Read the model definition and answer for the solid it produces. Units are mm, in the model's axes. Face numbers are marked on the shaded views. Give positions to 0.01 mm unless a question says otherwise; leave off trailing zeros. Put each result on its own line as item: value. Start each with the question number.
1. Given pin 1 Ø5 at (x, z) = (-13.5, -45.5) entering from +Y; pin 2 Ø10 at (x, z) = (2, -15.5) entering from -Y; pin 3 Ø1.5 at (x, y) = (-6.5, -9) entering from -Z; pin 4 Ø1 at (x, y) = (-8, -5.5) entering from -Z, each flat-ended and moving along its own axis, determine where each tip first touches the part or whether it passes through.
2. For a pull along Z with two mould halves and no side action, classify the marked faces 1, 2 and 3 as released by +Z, released by -Z, zero draft, split by the parting line, or undercut.
3. Consider L1, parallel to Z at x = 0, y = -8.5; L2, parallel to Z at x = 0, y = -1.85; L3, parallel to Z at x = 0, y = -11.25. Determine where each line is inside the solid, lowest interval first. Write a range as from..to.
4. A cutting plane is placed at A-A, the plane y = -9. Count the separate pieces of the cut face and the enclosed holes in it, plus the area to 3 significant figures.
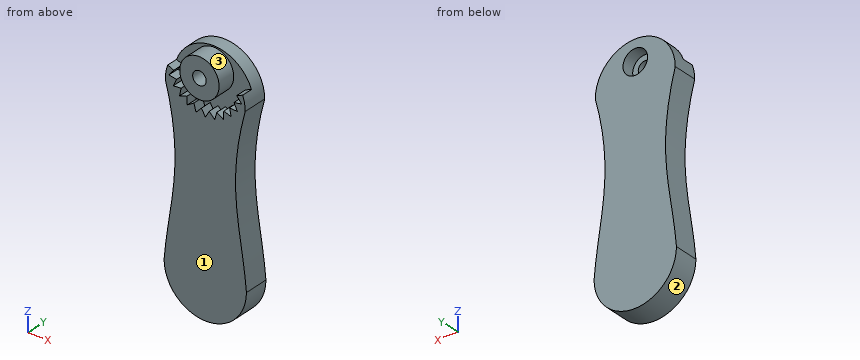
```python
from build123d import *

# Parameters (mm, degrees)
F1_DEPTH = 10.16
F2_R     = 8.128
F2_R_2   = 2.794
F3_DEPTH = 3.048
F4_DEPTH = 50.8
F5_R     = 8.128
F6_DEPTH = 4.572
F7_R     = 5.08
F7_R_2   = 2.794
F8_DEPTH = 5.08


with BuildPart() as f1:
    # F0 (on Front) → F1 (new body)
    with BuildSketch(Plane.XZ):
        with BuildLine():
            add(Edge.make_bspline(
                [(16.51, 16.2022389048), (8.1950903917, -14.7107664531), (15.1309384414, -29.2677398155), (17.018, -51.8697610952)],
                knots=[0, 0, 0, 0, 68.073895496, 68.073895496, 68.073895496, 68.073895496], degree=3))
            ThreePointArc((16.51, 16.2022389048), (0, 32.7122389048), (-16.51, 16.2022389048))
            add(Edge.make_bspline(
                [(-16.51, 16.2022389048), (-8.1950903917, -14.7107664531), (-15.1309384414, -29.2677398155), (-17.018, -51.8697610952)],
                knots=[0, 0, 0, 0, 68.073895496, 68.073895496, 68.073895496, 68.073895496], degree=3))
            ThreePointArc((-17.018, -51.8697610952), (0, -68.8877610952), (17.018, -51.8697610952))
        make_face()
    extrude(amount=F1_DEPTH)

    # F2 (on face) → F3 (join)
    with BuildSketch(Plane.XZ.offset(10.16)):
        with Locations((0, 24.0762389048)):
            Circle(F2_R)
        with Locations((0, 24.0762389048)):
            Circle(F2_R_2, mode=Mode.SUBTRACT)
    extrude(amount=F3_DEPTH)

    # F4 (cut, symmetric): a face of the model
    f4_faces = [f1.faces().sort_by_distance(p)[0] for p in [
        (0, -10.16, 24.0762389048),
    ]]
    extrude(f4_faces, amount=F4_DEPTH, both=True, mode=Mode.SUBTRACT)

    # F5 (on face) → F6 (cut)
    with BuildSketch(Plane.XZ.offset(10.16)):
        with BuildLine():
            ThreePointArc((15.469928865, 21.9695087018), (-0.0442530739, 32.7121795972), (-15.5006234178, 21.8864955545))
            Line((-15.5006234178, 21.8864955545), (-12.9936152173, 20.8281131752))
            Line((-12.9936152173, 20.8281131752), (-15.0273981388, 18.3203464733))
            Line((-15.0273981388, 18.3203464733), (-11.8387170074, 17.8129221485))
            Line((-11.8387170074, 17.8129221485), (-13.2132540393, 14.8913104783))
            Line((-13.2132540393, 14.8913104783), (-9.995795597, 15.1617323254))
            Line((-9.995795597, 15.1617323254), (-10.6312036432, 11.9960691377))
            Line((-10.6312036432, 11.9960691377), (-7.5719548797, 13.0286212217))
            Line((-7.5719548797, 13.0286212217), (-7.4313063342, 9.8028833542))
            Line((-7.4313063342, 9.8028833542), (-4.7080596678, 11.5375575014))
            Line((-4.7080596678, 11.5375575014), (-3.7995285128, 8.4392131139))
            Line((-3.7995285128, 8.4392131139), (-1.570549141, 10.7751963679))
            Line((-1.570549141, 10.7751963679), (0.0530640951, 7.9843099742))
            Line((0.0530640951, 7.9843099742), (1.6582359931, 10.7858434794))
            Line((1.6582359931, 10.7858434794), (3.9025728106, 8.4646112522))
            Line((3.9025728106, 8.4646112522), (4.7906504787, 11.5688800644))
            Line((4.7906504787, 11.5688800644), (7.5252781797, 9.8522035834))
            Line((7.5252781797, 9.8522035834), (7.6446497718, 13.0787988828))
            Line((7.6446497718, 13.0787988828), (10.7106417342, 12.0664451452))
            Line((10.7106417342, 12.0664451452), (10.0543698074, 15.2278489412))
            Line((10.0543698074, 15.2278489412), (13.2735417227, 14.9786522665))
            Line((13.2735417227, 14.9786522665), (11.8797664159, 17.8911352617))
            Line((11.8797664159, 17.8911352617), (15.0650317137, 18.4195780548))
            Line((15.0650317137, 18.4195780548), (13.0147541814, 20.913877324))
            Line((13.0147541814, 20.913877324), (15.469928865, 21.9695087018))
        make_face()
        with BuildLine():
            Line((-11.7664292563, 17.8014187834), (-11.8387170074, 17.8129221485))
            Line((-11.8387170074, 17.8129221485), (-11.8075561021, 17.8791554056))
            ThreePointArc((-11.8075561021, 17.8791554056), (-11.7870567643, 17.84025319), (-11.7664292563, 17.8014187834))
        make_face(mode=Mode.SUBTRACT)
        with BuildLine():
            Line((-9.9228554611, 15.1678628183), (-9.995795597, 15.1617323254))
            Line((-9.995795597, 15.1617323254), (-9.9813908269, 15.2334982572))
            ThreePointArc((-9.9813908269, 15.2334982572), (-9.952177253, 15.2006322819), (-9.9228554611, 15.1678628183))
        make_face(mode=Mode.SUBTRACT)
        with BuildLine():
            Line((-12.9261809524, 20.7996444858), (-12.9936152173, 20.8281131752))
            Line((-12.9936152173, 20.8281131752), (-12.9475091354, 20.8849645215))
            ThreePointArc((-12.9475091354, 20.8849645215), (-12.9369153807, 20.842286921), (-12.9261809524, 20.7996444858))
        make_face(mode=Mode.SUBTRACT)
        with BuildLine():
            Line((-7.5026013746, 13.0520292908), (-7.5719548797, 13.0286212217))
            Line((-7.5719548797, 13.0286212217), (-7.5751433977, 13.1017490531))
            ThreePointArc((-7.5751433977, 13.1017490531), (-7.5389133745, 13.0768293692), (-7.5026013746, 13.0520292908))
        make_face(mode=Mode.SUBTRACT)
        with BuildLine():
            Line((-4.646323367, 11.5768827546), (-4.7080596678, 11.5375575014))
            Line((-4.7080596678, 11.5375575014), (-4.7286561687, 11.6077973086))
            ThreePointArc((-4.7286561687, 11.6077973086), (-4.6875152535, 11.5922721575), (-4.646323367, 11.5768827546))
        make_face(mode=Mode.SUBTRACT)
        with BuildLine():
            Line((-1.5200179341, 10.8281533646), (-1.570549141, 10.7751963679))
            Line((-1.570549141, 10.7751963679), (-1.6073566312, 10.8384660687))
            ThreePointArc((-1.6073566312, 10.8384660687), (-1.5636957843, 10.8332377157), (-1.5200179341, 10.8281533646))
        make_face(mode=Mode.SUBTRACT)
        with BuildLine():
            Line((1.6946254161, 10.8493545514), (1.6582359931, 10.7858434794))
            Line((1.6582359931, 10.7858434794), (1.6073566312, 10.8384660687))
            ThreePointArc((1.6073566312, 10.8384660687), (1.651, 10.8438383667), (1.6946254161, 10.8493545514))
        make_face(mode=Mode.SUBTRACT)
        with BuildLine():
            Line((4.8107832969, 11.639254179), (4.7906504787, 11.5688800644))
            Line((4.7906504787, 11.5688800644), (4.7286561687, 11.6077973086))
            ThreePointArc((4.7286561687, 11.6077973086), (4.7697456655, 11.6234580392), (4.8107832969, 11.639254179))
        make_face(mode=Mode.SUBTRACT)
        with BuildLine():
            Line((7.6473559389, 13.1519461522), (7.6446497718, 13.0787988828))
            Line((7.6446497718, 13.0787988828), (7.5751433977, 13.1017490531))
            ThreePointArc((7.5751433977, 13.1017490531), (7.6112910502, 13.1267880715), (7.6473559389, 13.1519461522))
        make_face(mode=Mode.SUBTRACT)
        with Locations((0, 24.0762389048)):
            Circle(F5_R, mode=Mode.SUBTRACT)
        with BuildLine():
            Line((11.8481693767, 17.9571615707), (11.8797664159, 17.8911352617))
            Line((11.8797664159, 17.8911352617), (11.8075561021, 17.8791554056))
            ThreePointArc((11.8075561021, 17.8791554056), (11.8279270467, 17.9181250071), (11.8481693767, 17.9571615707))
        make_face(mode=Mode.SUBTRACT)
        with BuildLine():
            Line((12.9682741648, 20.9704233621), (13.0147541814, 20.913877324))
            Line((13.0147541814, 20.913877324), (12.9475091354, 20.8849645215))
            ThreePointArc((12.9475091354, 20.8849645215), (12.9579621013, 20.9276768234), (12.9682741648, 20.9704233621))
        make_face(mode=Mode.SUBTRACT)
        with BuildLine():
            Line((-12.9475091354, 20.8849645215), (-12.9936152173, 20.8281131752))
            Line((-12.9936152173, 20.8281131752), (-12.9261809524, 20.7996444858))
            ThreePointArc((-12.9261809524, 20.7996444858), (-12.9369153807, 20.842286921), (-12.9475091354, 20.8849645215))
        make_face()
        with BuildLine():
            Line((-11.8075561021, 17.8791554056), (-11.8387170074, 17.8129221485))
            Line((-11.8387170074, 17.8129221485), (-11.7664292563, 17.8014187834))
            ThreePointArc((-11.7664292563, 17.8014187834), (-11.7870567643, 17.84025319), (-11.8075561021, 17.8791554056))
        make_face()
        with BuildLine():
            Line((-9.9813908269, 15.2334982572), (-9.995795597, 15.1617323254))
            Line((-9.995795597, 15.1617323254), (-9.9228554611, 15.1678628183))
            ThreePointArc((-9.9228554611, 15.1678628183), (-9.952177253, 15.2006322819), (-9.9813908269, 15.2334982572))
        make_face()
        with BuildLine():
            Line((-7.5751433977, 13.1017490531), (-7.5719548797, 13.0286212217))
            Line((-7.5719548797, 13.0286212217), (-7.5026013746, 13.0520292908))
            ThreePointArc((-7.5026013746, 13.0520292908), (-7.5389133745, 13.0768293692), (-7.5751433977, 13.1017490531))
        make_face()
        with BuildLine():
            Line((-4.7286561687, 11.6077973086), (-4.7080596678, 11.5375575014))
            Line((-4.7080596678, 11.5375575014), (-4.646323367, 11.5768827546))
            ThreePointArc((-4.646323367, 11.5768827546), (-4.6875152535, 11.5922721575), (-4.7286561687, 11.6077973086))
        make_face()
        with BuildLine():
            Line((-1.6073566312, 10.8384660687), (-1.570549141, 10.7751963679))
            Line((-1.570549141, 10.7751963679), (-1.5200179341, 10.8281533646))
            ThreePointArc((-1.5200179341, 10.8281533646), (-1.5636957843, 10.8332377157), (-1.6073566312, 10.8384660687))
        make_face()
        with BuildLine():
            Line((1.6073566312, 10.8384660687), (1.6582359931, 10.7858434794))
            Line((1.6582359931, 10.7858434794), (1.6946254161, 10.8493545514))
            ThreePointArc((1.6946254161, 10.8493545514), (1.651, 10.8438383667), (1.6073566312, 10.8384660687))
        make_face()
        with BuildLine():
            Line((4.7286561687, 11.6077973086), (4.7906504787, 11.5688800644))
            Line((4.7906504787, 11.5688800644), (4.8107832969, 11.639254179))
            ThreePointArc((4.8107832969, 11.639254179), (4.7697456655, 11.6234580392), (4.7286561687, 11.6077973086))
        make_face()
        with BuildLine():
            Line((7.5751433977, 13.1017490531), (7.6446497718, 13.0787988828))
            Line((7.6446497718, 13.0787988828), (7.6473559389, 13.1519461522))
            ThreePointArc((7.6473559389, 13.1519461522), (7.6112910502, 13.1267880715), (7.5751433977, 13.1017490531))
        make_face()
        with BuildLine():
            Line((11.8075561021, 17.8791554056), (11.8797664159, 17.8911352617))
            Line((11.8797664159, 17.8911352617), (11.8481693767, 17.9571615707))
            ThreePointArc((11.8481693767, 17.9571615707), (11.8279270467, 17.9181250071), (11.8075561021, 17.8791554056))
        make_face()
        with BuildLine():
            Line((12.9475091354, 20.8849645215), (13.0147541814, 20.913877324))
            Line((13.0147541814, 20.913877324), (12.9682741648, 20.9704233621))
            ThreePointArc((12.9682741648, 20.9704233621), (12.9579621013, 20.9276768234), (12.9475091354, 20.8849645215))
        make_face()
    extrude(amount=-F6_DEPTH, mode=Mode.SUBTRACT)

    # F7 (on face) → F8 (cut)
    with BuildSketch(Plane(origin=(0, 0, 0), x_dir=(-1, 0, 0), z_dir=(0, 1, 0))):
        with Locations((0, 24.0762389048)):
            Circle(F7_R)
        with Locations((0, 24.0762389048)):
            Circle(F7_R_2, mode=Mode.SUBTRACT)
        with Locations((0, 24.0762389048)):
            Circle(F7_R_2)
    extrude(amount=-F8_DEPTH, mode=Mode.SUBTRACT)


solid = f1.part
```
Return value:
1. pin 1: stops at y = 0
1. pin 2: stops at y = -10.16
1. pin 3: stops at z = -67.89
1. pin 4: stops at z = -67.15
2. face 1: zero draft
2. face 2: released by -Z
2. face 3: undercut
3. L1: z = -68.89..8.08, 15.95..21.28, 26.87..32.2
3. L2: z = -68.89..19, 29.16..32.71
3. L3: z = 15.95..21.28, 26.87..32.2
4. separate pieces: 2
4. enclosed holes: 1
4. area: 2,490 mm2
